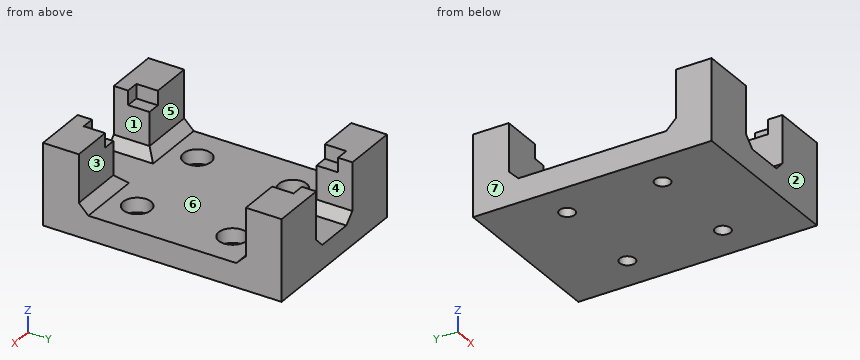
from build123d import *

# Parameters (mm, degrees)
SKETCH_W        = 35
SKETCH_H        = 50
PAD_DEPTH       = 5
SKETCH004_R     = 2.9
POCKET_DEPTH    = 3
SKETCH005_R     = 1.6
POCKET001_DEPTH = 5
SKETCH006_W     = 11.5
SKETCH006_H     = 7.5
PAD001_DEPTH    = 12
SKETCH007_W     = 17.5
SKETCH007_H     = 44
POCKET002_DEPTH = 3
CHAMFER_SIZE    = 2


with BuildPart() as part:
    # Sketch → Pad (new body)
    with BuildSketch(Plane.XY):
        with Locations((17.5, 25)):
            Rectangle(SKETCH_W, SKETCH_H)
    extrude(amount=PAD_DEPTH)

    # Sketch004 → Pocket (cut)
    with BuildSketch(Plane.XY.offset(5)):
        with Locations((7.5, 15)):
            Circle(SKETCH004_R)
        with Locations((7.5, 35)):
            Circle(SKETCH004_R)
        with Locations((27.5, 15)):
            Circle(SKETCH004_R)
        with Locations((27.5, 35)):
            Circle(SKETCH004_R)
    extrude(amount=-POCKET_DEPTH, mode=Mode.SUBTRACT)

    # Sketch005 → Pocket001 (cut)
    with BuildSketch(Plane.XY.offset(2)):
        with Locations((7.5, 15)):
            Circle(SKETCH005_R)
        with Locations((7.5, 35)):
            Circle(SKETCH005_R)
        with Locations((27.5, 15)):
            Circle(SKETCH005_R)
        with Locations((27.5, 35)):
            Circle(SKETCH005_R)
    extrude(amount=-POCKET001_DEPTH, mode=Mode.SUBTRACT)

    # Sketch006 → Pad001 (new body)
    with BuildSketch(Plane.XY.offset(5)):
        with Locations((5.75, 3.75)):
            Rectangle(SKETCH006_W, SKETCH006_H)
        with Locations((5.75, 46.25)):
            Rectangle(SKETCH006_W, SKETCH006_H)
        with Locations((29.25, 3.75)):
            Rectangle(SKETCH006_W, SKETCH006_H)
        with Locations((29.25, 46.25)):
            Rectangle(SKETCH006_W, SKETCH006_H)
    extrude(amount=PAD001_DEPTH)

    # Sketch007 → Pocket002 (cut)
    with BuildSketch(Plane.XY.offset(17)):
        with Locations((17.5, 25)):
            Rectangle(SKETCH007_W, SKETCH007_H)
    extrude(amount=-POCKET002_DEPTH, mode=Mode.SUBTRACT)

    # Chamfer
    chamfer_edges = [part.edges().sort_by_distance(p)[0] for p in [
        (5.75, 7.5, 5),
        (11.5, 3.75, 5),
        (29.25, 7.5, 5),
        (23.5, 3.75, 5),
        (5.75, 42.5, 5),
        (11.5, 46.25, 5),
        (29.25, 42.5, 5),
        (23.5, 46.25, 5),
    ]]
    chamfer(chamfer_edges, length=CHAMFER_SIZE)


solid = part.part
The model under review builds one solid part; all positions refer to its coordinate system, in mm. Face numbers are marked on the shaded views. A direction names the side the tool comes from. Give positions to 0.01 mm unless a question says otherwise; leave off trailing zeros. Write each loop counter-clockwise with the first axis right and the second up, starting at its lowest first coordinate (ties: lowest second). Pieces come first, ordered by that corner, then holes. Notation, with made-up numbers: M 61.25,85 L 66.25,85 A25 ccw 66.25,123 Z; hole C -4,-36 d10. An arc over 180 degrees is marked long. One line per question, with ' | ' between items. Start each with the question number.
Item 1: Wall thickness on line 1 (Y direction, x = 6, z = 12); line 2 (Y direction, x = 27.5, z = 3); line 3 (X direction, y = 44.5, z = 15.25): over which ranges is each line inside the solid? List them lowest first. Write a range as from..to.
Item 2: We need section B-B on z = 11.75. Write out the cut boundary in (x, y), plus the area to 3 significant figures.
Item 3: We need section D-D on z = 3.75. Write out the cut boundary in (x, y).
Item 4: Draft analysis for pull direction Y (two halves, no side actions). For the marked faces 1, 2 and 3, state which applies: released by +Y, released by -Y, zero draft, split by the parting line, or undercut.
Item 5: We need section C-C on y = 35. Write out the cut boundary in (x, z).
Item 6: We need section A-A on x = 27.5. Write out the cut boundary in (y, z), plus the area to 3 significant figures.
Item 7: For pin 1 (5 mm diameter, centred on x = 7.5, y = 15, fed in from +Z); pin 2 (5 mm diameter, centred on x = 26, y = 29, fed in from +Z); pin 3 (8 mm diameter, centred on x = 31.5, z = 12.5, fed in from -Y); pin 4 (10 mm diameter, centred on x = 14, y = 11, fed in from +Z), all flat-tipped, find the tip position at first contact; note any pin that passes through.
Item 8: For the marked faces 4, 5, 6 and 7, list the 3-axis set-ups (+Z, -Z, +X, -X, +Y, -Y) from which the entire face can be reached by the end or side of a thin tool; tool diameter is ignored.
Results found:
1) line 1: y = 0..7.5, 42.5..50 | line 2: y = 0..12.1, 17.9..32.1, 37.9..50 | line 3: x = 0..8.75, 26.25..35
2) outline: M 0,0 L 11.5,0 L 11.5,7.5 L 0,7.5 Z; M 0,42.5 L 11.5,42.5 L 11.5,50 L 0,50 Z; M 23.5,0 L 35,0 L 35,7.5 L 23.5,7.5 Z; M 23.5,42.5 L 35,42.5 L 35,50 L 23.5,50 Z | area: 345 mm2
3) outline: M 0,0 L 35,0 L 35,50 L 0,50 Z; hole C 7.5,15 d5.8; hole C 7.5,35 d5.8; hole C 27.5,15 d5.8; hole C 27.5,35 d5.8
4) face 1: zero draft | face 2: released by -Y | face 3: undercut
5) outline: M 0,0 L 5.9,0 L 5.9,2 L 4.6,2 L 4.6,5 L 0,5 Z; M 9.1,0 L 25.9,0 L 25.9,2 L 24.6,2 L 24.6,5 L 10.4,5 L 10.4,2 L 9.1,2 Z; M 29.1,0 L 35,0 L 35,5 L 30.4,5 L 30.4,2 L 29.1,2 Z
6) outline: M 0,0 L 13.4,0 L 13.4,2 L 12.1,2 L 12.1,5 L 9.5,5 L 7.5,7 L 7.5,17 L 0,17 Z; M 16.6,0 L 33.4,0 L 33.4,2 L 32.1,2 L 32.1,5 L 17.9,5 L 17.9,2 L 16.6,2 Z; M 36.6,0 L 50,0 L 50,17 L 42.5,17 L 42.5,7 L 40.5,5 L 37.9,5 L 37.9,2 L 36.6,2 Z | area: 386 mm2
7) pin 1: stops at z = 2 | pin 2: stops at z = 5 | pin 3: stops at y = 0 | pin 4: stops at z = 14
8) face 4: +Z, +Y, -Y | face 5: +Z, +X, -X | face 6: +Z | face 7: +Z, -Z, -X, +Y, -Y
